```python
from build123d import *

# Parameters (mm, degrees)
ESQUISSE1_R        = 31.5
ESQUISSE1_R_2      = 29.5
BOSS_EXTRU_1_DEPTH = 160
ESQUISSE2_R        = 30
BOSS_EXTRU_2_DEPTH = 5
ESQUISSE3_R        = 30
BOSS_EXTRU_3_DEPTH = 5


with BuildPart() as part:
    # Esquisse1 → Boss.-Extru.1 (new body)
    with BuildSketch(Plane.XY):
        Circle(ESQUISSE1_R)
        Circle(ESQUISSE1_R_2, mode=Mode.SUBTRACT)
    extrude(amount=BOSS_EXTRU_1_DEPTH)

    # Esquisse2 → Boss.-Extru.2 (add)
    with BuildSketch(Plane(origin=(0, 0, 1), x_dir=(-1, 0, 0), z_dir=(0, 0, -1))):
        Circle(ESQUISSE2_R)
    extrude(amount=-BOSS_EXTRU_2_DEPTH)

    # Esquisse3 → Boss.-Extru.3 (add)
    with BuildSketch(Plane.XY.offset(159)):
        Circle(ESQUISSE3_R)
    extrude(amount=-BOSS_EXTRU_3_DEPTH)


solid = part.part
```
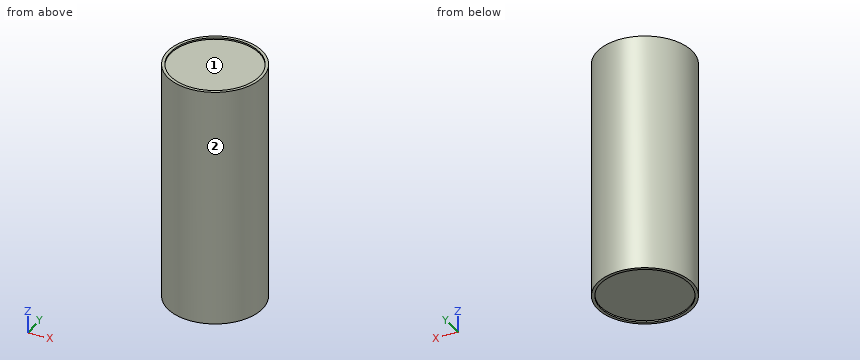
The listing builds one solid part. Answer for the finished solid, in the listing's coordinates (mm). Face numbers are marked on the shaded views. Coordinates: 2 decimals unless noted, no trailing zeros. Write each loop counter-clockwise with the first axis right and the second up, starting at its lowest first coordinate (ties: lowest second). Pieces come first, ordered by that corner, then holes. Notation, with made-up numbers: (34.25, -20.5) - (54.25, -20.5) arc R14 cw to (54.25, -15.5) - close; hole circle Ø10 at (83.5, 23.25). An arc over 180 degrees is marked (long way). One line per item, written item: value.
1) Consider line 1 along Y through (x, z) = (0, 0.25); line 2 along Z through (x, y) = (-7, 13.5); line 3 along X through (y, z) = (1, 42.5). Determine where each line is inside the solid, lowest interval first. Write a range as from..to.
Geometry check:
line 1: y = -31.5..-29.5, 29.5..31.5
line 2: z = 1..6, 154..159
line 3: x = -31.48..-29.48, 29.48..31.48
2) For a pull along Y with two mould halves and no side action, classify the marked faces 1 and 2 as pulls with the +Y half, pulls with the -Y half, needs draft (parallel to the pull), parting line crosses it, or undercut.
Geometry check:
face 1: undercut
face 2: parting line crosses it
3) Find section A-A (y = 0). Give the vertices of the cut face in (x, z), and give its area (3 significant figures).
Geometry check:
outline: (-31.5, 0) - (-29.5, 0) - (-29.5, 1) - (29.5, 1) - (29.5, 0) - (31.5, 0) - (31.5, 160) - (29.5, 160) - (29.5, 159) - (-29.5, 159) - (-29.5, 160) - (-31.5, 160) - close; hole (-29.5, 6) - (29.5, 6) - (29.5, 154) - (-29.5, 154) - close
area: 1,230 mm2
4) Each of these flat-tipped pins is pushed along its axis until it touches: pin 1 Ø6 at (x, z) = (1, 127.5) entering from -Y; pin 2 Ø5 at (x, y) = (-3.5, -7.5) entering from +Z; pin 3 Ø6 at (x, z) = (2.5, 52) entering from +Y. Where does it stop, or does it pass through?
Geometry check:
pin 1: stops at y = -31.5
pin 2: stops at z = 159
pin 3: stops at y = 31.5
5) Find section C-C (z = 86). Give the vertices of the cut face in (x, y).
Geometry check:
outline: circle Ø63 at (0, 0); hole circle Ø59 at (0, 0)
